Design review of the part built by this model. Coordinates are the model's own, in mm. Face numbers are marked on the shaded views. A direction names the side the tool comes from. Coordinates: 2 decimals unless noted, no trailing zeros. Write each loop counter-clockwise with the first axis right and the second up, starting at its lowest first coordinate (ties: lowest second). Pieces come first, ordered by that corner, then holes. Notation, with made-up numbers: (-19.75, 14.25) - (5.25, 14.25) arc R28 cw to (5.25, 46.25) - close; hole circle Ø10 at (12.5, 22). An arc over 180 degrees is marked (long way). Answer as CSV lines item,"result". Start each with the question number.
Q1. We need section A-A (y = 11.43). Write out the cut boundary in (x, z), plus the area to 3 significant figures.
Q2. We need section C-C (x = 40.5). Write out the cut boundary in (y, z).
Q3. We need section B-B (y = 28). Write out the cut boundary in (x, z), plus the area to 3 significant figures.
Q4. Mouldability with a two-part tool opening along X and no side actions: class the marked faces 4, 5, 6 and 7 as pulls with the +X half, pulls with the -X half, needs draft (parallel to the pull), parting line crosses it, or undercut.
Q5. Machinability: for the marked faces 1, 2 and 3, which of the approach directions +Z, -Z, +X, -X, +Y, -Y give a long, thin tool a straight path to every point of the face, cutting with its end or side? Answer none if there is none.
Q6. Clearance check with flat-ended pins moving along their axes: pin 1 (5 mm diameter, centred on x = -6.1, z = 5.78, fed in from +Y); pin 2 (6 mm diameter, centred on y = 42.418, z = 11.938, fed in from +X); pin 3 (1.5 mm diameter, centred on y = 17.5, z = 8.5, fed in from -X). State where each tip first meets the part, or that it passes through.
Q7. For line 1 along Z through (x, y) = (0.2, 11.43); line 2 along X through (y, z) = (44, 15); line 3 along Y through (x, z) = (-7, 17.75), list the stretches that pass through material, from the lowest coordinate up. Write a range as [from, to].
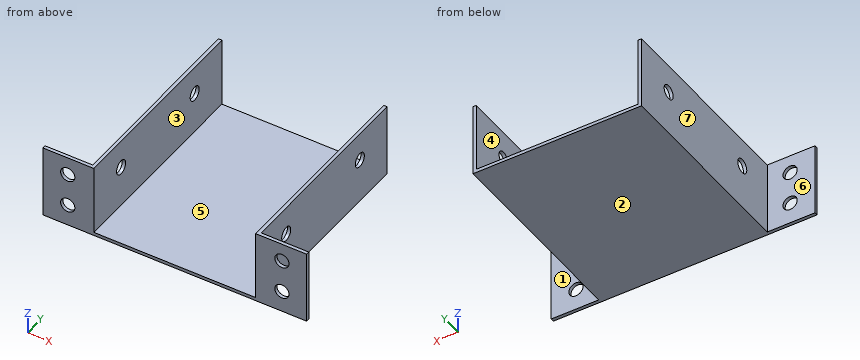
from build123d import *

# Parameters (mm, degrees)
F0_W     = 44.958
F0_H     = 53.848
F1_DEPTH = 0.889
F2_W     = 0.889
F2_H     = 18.669
F3_DEPTH = 53.848
F4_W     = 0.889
F4_H     = 19.558
F5_DEPTH = 12.7
F6_W     = 0.889
F6_H     = 19.558
F7_DEPTH = 12.7
F9_D     = 3.7973
F11_D    = 3.7973


# Not quite as in the source:
# - a feature names something its author has since deleted; it is built from what else it names


with BuildPart() as f1:
    # F0 (on Top) → F1 (new body)
    with BuildSketch(Plane.XY):
        with Locations((22.479, 26.924)):
            Rectangle(F0_W, F0_H)
    extrude(amount=F1_DEPTH)

    # F2 (on face) → F3 (join, through all)
    with BuildSketch(Plane.XZ):
        with Locations((0.4445, 10.2235)):
            Rectangle(F2_W, F2_H)
        with Locations((44.5135, 10.2235)):
            Rectangle(F2_W, F2_H)
    extrude(amount=-F3_DEPTH)

    # F4 (on face) → F5 (join)
    with BuildSketch(Plane(origin=(0, 0, 0), x_dir=(0, -1, 0), z_dir=(-1, 0, 0))):
        with Locations((-0.4445, 9.779)):
            Rectangle(F4_W, F4_H)
    extrude(amount=F5_DEPTH)

    # F6 (on face) → F7 (join)
    with BuildSketch(Plane.YZ.offset(44.958)):
        with Locations((0.4445, 9.779)):
            Rectangle(F6_W, F6_H)
    extrude(amount=F7_DEPTH)

    # F9 (through all)
    with Locations(Plane.XZ):
        with Locations((-6.096, 14.6685), (-6.096, 5.7785), (51.054, 5.7785), (51.054, 14.6685)):
            Hole(F9_D / 2)

    # F11 (through all)
    with Locations(Plane(origin=(0, 0, 0), x_dir=(0, -1, 0), z_dir=(-1, 0, 0))):
        with Locations((-11.43, 11.938), (-42.418, 11.938)):
            Hole(F11_D / 2)


solid = f1.part
Results list:
1,outline,"(0, 0) - (44.96, 0) - (44.96, 10.04) - (44.07, 10.04) - (44.07, 0.89) - (0.89, 0.89) - (0.89, 10.04) - (0, 10.04) - close; (0, 13.84) - (0.89, 13.84) - (0.89, 19.56) - (0, 19.56) - close; (44.07, 13.84) - (44.96, 13.84) - (44.96, 19.56) - (44.07, 19.56) - close"
1,area,"66.4 mm2"
2,outline,"(0, 0) - (53.85, 0) - (53.85, 0.89) - (0, 0.89) - close"
3,outline,"(0, 0) - (44.96, 0) - (44.96, 19.56) - (44.07, 19.56) - (44.07, 0.89) - (0.89, 0.89) - (0.89, 19.56) - (0, 19.56) - close"
3,area,"73.2 mm2"
4,face 4,"undercut"
4,face 5,"undercut"
4,face 6,"needs draft"
4,face 7,"pulls with the -X half"
5,face 1,"+Z, -Z, +X, +Y"
5,face 2,"-Z, +X, -X, +Y, -Y"
5,face 3,"+Z, +Y, -Y"
6,pin 1,"stops at y = 0.89"
6,pin 2,"stops at x = 44.96"
6,pin 3,"stops at x = 0"
7,line 1,"z = [0, 10.04], [13.84, 19.56]"
7,line 2,"x = [0, 0.89], [44.07, 44.96]"
7,line 3,"y = [0, 0.89]"
